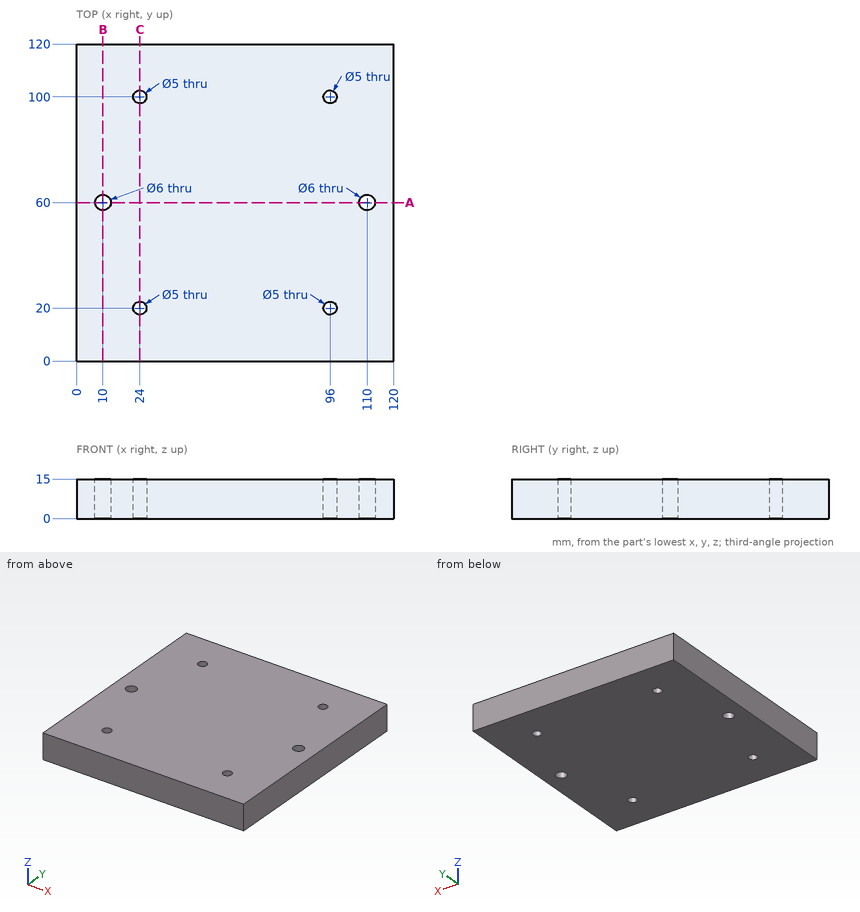
Here's the drawing with two shaded views (mm, measured from the low corner). I have some questions. Coordinates: 2 decimals unless noted, no trailing zeros. Order: outer loops, then holes, each group sorted by start corner. A loop starts at its lowest first (then second) coordinate and runs counter-clockwise, first axis right, second up. Notation, with made-up numbers: (24.5, 31.5) -> (74.5, 31.5) arc R24 cw to (74.5, 60.5) -> close; hole circle Ø6 at (60.5, 23.25). An arc over 180 degrees is marked (long way). One line per question, with ' | ' between items.
Q1. I'm going to push a flat-ended pin straight in: P1, Ø4.5, axis at x = 24, y = 100, coming from the -Z side. Where does the tip first touch, or does it pass through?
Return value:
P1: through
Q2. Imagine slicing it at C-C on x = 24. Please give me the cut outline in (y, z).
Return value:
outline: (0, 0) -> (17.5, 0) -> (17.5, 15) -> (0, 15) -> close; (22.5, 0) -> (97.5, 0) -> (97.5, 15) -> (22.5, 15) -> close; (102.5, 0) -> (120, 0) -> (120, 15) -> (102.5, 15) -> close
Q3. If I drill on L1, parallel to Y at x = 24, z = 9; L2, parallel to X at y = 100, z = 5.75; L3, parallel to X at y = 22, z = 14.25, over which ranges is the centre line in solid material (lowest first)?
Return value:
L1: 0 to 17.5, 22.5 to 97.5, 102.5 to 120 | L2: 0 to 21.5, 26.5 to 93.5, 98.5 to 120 | L3: 0 to 22.5, 25.5 to 94.5, 97.5 to 120
Q4. Imagine slicing it at A-A on y = 60. Please give me the cut outline in (x, z).
Return value:
outline: (0, 0) -> (7, 0) -> (7, 15) -> (0, 15) -> close; (13, 0) -> (107, 0) -> (107, 15) -> (13, 15) -> close; (113, 0) -> (120, 0) -> (120, 15) -> (113, 15) -> close
Q5. Imagine slicing it at B-B on x = 10. Please give me the cut outline in (y, z), and give its area (3 significant figures).
Return value:
outline: (0, 0) -> (57, 0) -> (57, 15) -> (0, 15) -> close; (63, 0) -> (120, 0) -> (120, 15) -> (63, 15) -> close | area: 1,710 mm²
